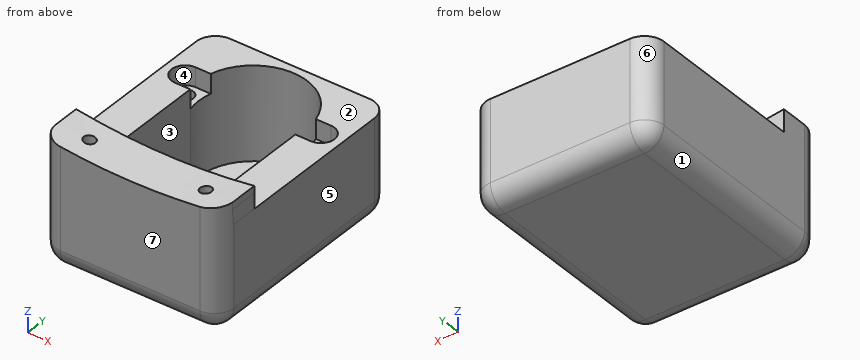
from build123d import *

# Parameters (mm, degrees)
ESQUISSE1_W             = 26
ESQUISSE1_H             = 46
BOSS_EXTRU_1_DEPTH      = 10
ESQUISSE1_5_W           = 26
ESQUISSE1_5_H           = 46
BOSS_EXTRU_2_DEPTH      = 48
ESQUISSE2_R             = 14
ESQUISSE2_R_2           = 2.5
ENL_V_MAT_EXTRU_1_DEPTH = 24
ESQUISSE2_17_R          = 2.1
ENL_V_MAT_EXTRU_2_DEPTH = 5
ESQUISSE2_18_R          = 2.1
ENL_V_MAT_EXTRU_3_DEPTH = 14
BOSS_EXTRU_7_DEPTH      = 12
CONG_1_R                = 5
CONG_2_R                = 5
ESQUISSE6_R             = 1.5
ENL_V_MAT_EXTRU_4_DEPTH = 174


with BuildPart() as part:
    # Esquisse1 → Boss.-Extru.1 (new body)
    with BuildSketch(Plane(origin=(0, 0, 0), x_dir=(0, 0, -1), z_dir=(0, 1, 0))):
        with Locations((171, 0)):
            Rectangle(ESQUISSE1_W, ESQUISSE1_H)
    extrude(amount=BOSS_EXTRU_1_DEPTH)

    # Esquisse1<5> → Boss.-Extru.2 (add)
    with BuildSketch(Plane(origin=(0, 0, 0), x_dir=(0, 0, -1), z_dir=(0, 1, 0))):
        with Locations((171, 0)):
            Rectangle(ESQUISSE1_5_W, ESQUISSE1_5_H)
    extrude(amount=-BOSS_EXTRU_2_DEPTH)

    # Esquisse2 → Enlèv. mat.-Extru.1 (cut)
    # profile 1 of 3: a face of its own
    with BuildSketch(Plane.XY.offset(-158)):
        with Locations((0, -6)):
            Circle(ESQUISSE2_R)
        with Locations((0, 2)):
            Circle(ESQUISSE2_R_2, mode=Mode.SUBTRACT)
    # profile 2 of 3: a face of its own
    with BuildSketch(Plane.XY.offset(-158)):
        with BuildLine():
            ThreePointArc((13.555441712, -9.5), (0, -20), (-13.555441712, -9.5))
            Line((-13.555441712, -9.5), (-13.555441712, -36))
            Line((-13.555441712, -36), (13.555441712, -36))
            Line((13.555441712, -36), (13.555441712, -9.5))
        make_face()
    # profile 3 of 3: a face of its own
    with BuildSketch(Plane.XY.offset(-158)):
        with Locations((0, 2)):
            Circle(ESQUISSE2_R_2)
    extrude(amount=-ENL_V_MAT_EXTRU_1_DEPTH, mode=Mode.SUBTRACT)

    # Esquisse2<17> → Enlèv. mat.-Extru.2 (cut)
    # profile 1 of 2: a face of its own
    with BuildSketch(Plane.XY.offset(-158)):
        with BuildLine():
            Line((-13.555441712, -2.5), (-17.5, -2.5))
            ThreePointArc((-17.5, -2.5), (-21, -6), (-17.5, -9.5))
            Line((-17.5, -9.5), (-13.555441712, -9.5))
            ThreePointArc((-13.555441712, -9.5), (-14, -6), (-13.555441712, -2.5))
        make_face()
        with Locations((-17.5, -6)):
            Circle(ESQUISSE2_17_R, mode=Mode.SUBTRACT)
    # profile 2 of 2: a face of its own
    with BuildSketch(Plane.XY.offset(-158)):
        with BuildLine():
            Line((17.5, -2.5), (13.555441712, -2.5))
            ThreePointArc((13.555441712, -2.5), (13.888415748, -4.235939905), (14, -6))
            ThreePointArc((14, -6), (13.888415748, -7.764060095), (13.555441712, -9.5))
            Line((13.555441712, -9.5), (17.5, -9.5))
            ThreePointArc((17.5, -9.5), (21, -6), (17.5, -2.5))
        make_face()
        with Locations((17.5, -6)):
            Circle(ESQUISSE2_17_R, mode=Mode.SUBTRACT)
    extrude(amount=-ENL_V_MAT_EXTRU_2_DEPTH, mode=Mode.SUBTRACT)

    # Esquisse2<18> → Enlèv. mat.-Extru.3 (cut)
    with BuildSketch(Plane.XY.offset(-158)):
        with Locations((-17.5, -6)):
            Circle(ESQUISSE2_18_R)
        with Locations((17.5, -6)):
            Circle(ESQUISSE2_18_R)
    extrude(amount=-ENL_V_MAT_EXTRU_3_DEPTH, mode=Mode.SUBTRACT)

    # Esquisse5 → Boss.-Extru.7 (add)
    with BuildSketch(Plane.XZ.offset(48)):
        with BuildLine():
            Line((-23, -158), (-23, -154))
            Line((-23, -154), (-23, -152.249792013))
            ThreePointArc((-23, -152.249792013), (-0.012314253, -153.999999501), (22.975654778, -152.253516723))
            Line((22.975654778, -152.253516723), (22.975654778, -154))
            Line((22.975654778, -154), (23, -158))
            Line((23, -158), (23, -184))
            Line((23, -184), (-23, -184))
            Line((-23, -184), (-23, -158))
        make_face()
    extrude(amount=-BOSS_EXTRU_7_DEPTH)

    # Congé1
    cong_1_edges = [part.edges().sort_by_distance(p)[0] for p in [
        (23, 10, -171),
        (0, 10, -184),
        (23, -19, -184),
    ]]
    fillet(cong_1_edges, radius=CONG_1_R)

    # Congé2
    # the kernel refuses this fillet: 5 mm, written as the material it takes off along each edge
    with BuildSketch(Plane(origin=(-18, -43, -179), x_dir=(-1, 0, 0), z_dir=(0, -1, 0))) as cong_2_piece_1_section:
        Polygon((0, 0), (CONG_2_R * 1.02, 0), (CONG_2_R * 1.02, CONG_2_R * 1.02), (0, CONG_2_R * 1.02), align=None)
    cong_2_piece_1 = extrude(amount=CONG_2_R * 1.02, mode=Mode.PRIVATE)
    cong_2_piece_1 = cong_2_piece_1 - Plane(origin=(-18, -43, -179), x_dir=(0.7071067811865475, 0, 0.7071067811865475), z_dir=(0, -1, 0)) * Sphere(CONG_2_R, mode=Mode.PRIVATE)
    add(cong_2_piece_1, mode=Mode.SUBTRACT)
    with BuildSketch(Plane(origin=(18, -48, -179), x_dir=(0, 0, -1), z_dir=(-1, 0, 0))) as cong_2_piece_2:
        with BuildLine():
            CenterArc((5 - CONG_2_R, -CONG_2_R), CONG_2_R, 0, 90)
            Line((5 - CONG_2_R, 0), (5, 0))
            Line((5, 0), (5, -CONG_2_R))
        make_face()
    revolve(axis=Axis((18, -48, -179), (0, -1, 0)), revolution_arc=90, mode=Mode.SUBTRACT)
    with BuildSketch(Plane(origin=(-23, 5, -179), x_dir=(0, 1, 0), z_dir=(0, 0, 1))) as cong_2_piece_3:
        with BuildLine():
            CenterArc((5 - CONG_2_R, -CONG_2_R), CONG_2_R, 0, 90)
            Line((5, -CONG_2_R), (5, 0))
            Line((5, 0), (5 - CONG_2_R, 0))
        make_face()
    revolve(axis=Axis((-23, 5, -179), (-1, 0, 0)), revolution_arc=90, mode=Mode.SUBTRACT)
    with BuildSketch(Plane(origin=(-23, -48, -179), x_dir=(0, 1, 0), z_dir=(0, 0, 1))) as cong_2_piece_4:
        with BuildLine():
            CenterArc((CONG_2_R, -CONG_2_R), CONG_2_R, 90, 90)
            Line((0, -CONG_2_R), (0, 0))
            Line((0, 0), (CONG_2_R, 0))
        make_face()
    extrude(amount=39.250207987, mode=Mode.SUBTRACT)
    with BuildSketch(Plane(origin=(23, -48, -145.5), x_dir=(0, 1, 0), z_dir=(0, 0, -1)), Plane(origin=(-23, 10, -179), x_dir=(1, 0, 0), z_dir=(0, 0, 1))) as cong_2_piece_5:
        with BuildLine():
            CenterArc((CONG_2_R, -CONG_2_R), CONG_2_R, 90, 90)
            Line((0, -CONG_2_R), (0, 0))
            Line((0, 0), (CONG_2_R, 0))
        make_face()
    extrude(amount=33.5, mode=Mode.SUBTRACT)
    with BuildSketch(Plane(origin=(18, -48, -184), x_dir=(0, 0, 1), z_dir=(-1, 0, 0))) as cong_2_piece_6:
        with BuildLine():
            CenterArc((CONG_2_R, CONG_2_R), CONG_2_R, 180, 90)
            Line((0, CONG_2_R), (0, 0))
            Line((0, 0), (CONG_2_R, 0))
        make_face()
    extrude(amount=36, mode=Mode.SUBTRACT)
    with BuildSketch(Plane(origin=(-23, 5, -184), x_dir=(0, 0, 1), z_dir=(0, -1, 0))) as cong_2_piece_7:
        with BuildLine():
            CenterArc((CONG_2_R, -CONG_2_R), CONG_2_R, 90, 90)
            Line((0, -CONG_2_R), (0, 0))
            Line((0, 0), (CONG_2_R, 0))
        make_face()
    extrude(amount=48, mode=Mode.SUBTRACT)

    # Esquisse6 → Enlèv. mat.-Extru.4 (cut)
    with BuildSketch(Plane.XY):
        with Locations((-15, -42)):
            Circle(ESQUISSE6_R)
        with Locations((15, -42)):
            Circle(ESQUISSE6_R)
    extrude(amount=-ENL_V_MAT_EXTRU_4_DEPTH, mode=Mode.SUBTRACT)


solid = part.part
Could you check a few things on this model? Use its own coordinates, in mm. Face numbers are marked on the shaded views. A direction names the side the tool comes from. Coordinates: 2 decimals unless noted, no trailing zeros. Loops run counter-clockwise (first coordinate to the right, second up) from the corner with the lowest first, then second, coordinate; pieces in that order, holes last.
1. Imagine slicing it at D-D (x = 0). Please give me the cut outline in (y, z), and give its area (3 significant figures).
2. Imagine slicing it at A-A (z = -160). Please give me the cut outline in (x, y), and give its area (3 significant figures).
3. Imagine slicing it at B-B (y = -21). Please give me the cut outline in (x, z).
4. Imagine slicing it at C-C (z = -178). Please give me the cut outline in (x, y).
5. For the marked faces 1, 2 and 3, which set-ups out of +Z, -Z, +X, -X, +Y, -Y let a thin tool reach every point of the face, with its end or its side?
6. For P1, Ø22.5, axis at x = -3.5, y = -9.5, coming from the +Z side; P2, Ø2.5, axis at x = -15.5, y = -42, coming from the +Z side; P3, Ø5.5, axis at x = 17.5, y = -6, coming from the +Z side, each with a flat end and sliding along its axis, tell me the tip position at first contact or that it passes through.
7. We'd pull the mould along X, two halves only. Please class the marked faces 4, 5, 6 and 7: released by +X, released by -X, zero draft, split by the parting line, or undercut.
8. I need wall thicknesses on L1, parallel to X at y = -42, z = -158.25; L2, parallel to Y at x = -15, z = -162.25; L3, parallel to X at y = -6, z = -175. Which ranges of each line are inside material? Lowest first, please.
Computed values:
1. outline: (-48, -179) arc R5 ccw to (-43, -184) - (5, -184) arc R5 ccw to (10, -179) - (10, -158) - (8, -158) - (8, -182) - (-36, -182) - (-36, -154) - (-48, -154) - close
1. area: 489 mm2
2. outline: (-23, -43) arc R5 ccw to (-18, -48) - (18, -48) arc R5 ccw to (23, -43) - (23, 5) arc R5 ccw to (18, 10) - (-18, 10) arc R5 ccw to (-23, 5) - close; hole (-17.5, -9.5) - (-13.56, -9.5) - (-13.56, -36) - (13.56, -36) - (13.56, -9.5) - (17.5, -9.5) arc R3.5 ccw to (17.5, -2.5) - (13.56, -2.5) arc R14 ccw to (-13.56, -2.5) - (-17.5, -2.5) arc R3.5 ccw to start; hole circle Ø3 at (-15, -42); hole circle Ø3 at (15, -42)
2. area: 1,420 mm2
3. outline: (-23, -179) arc R5 ccw to (-18, -184) - (18, -184) arc R5 ccw to (23, -179) - (23, -158) - (13.56, -158) - (13.56, -182) - (-13.56, -182) - (-13.56, -158) - (-23, -158) - close
4. outline: (-23, -43) arc R5 ccw to (-18, -48) - (18, -48) arc R5 ccw to (23, -43) - (23, 5) arc R5 ccw to (18, 10) - (-18, 10) arc R5 ccw to (-23, 5) - close; hole (-13.56, -36) - (13.56, -36) - (13.56, -9.5) arc R14 ccw (long way) to (-13.56, -9.5) - close
5. face 1: -Z, -X, +Y, -Y
5. face 2: +Z, +X, -X, +Y
5. face 3: +Z
6. P1: stops at z = -158
6. P2: stops at z = -153.07
6. P3: stops at z = -163
7. face 4: undercut
7. face 5: released by +X
7. face 6: released by -X
7. face 7: zero draft
8. L1: x = -23 to -16.5, -13.5 to 13.5, 16.5 to 23
8. L2: y = -48 to -43.5, -40.5 to -9.5, -2.5 to 10
8. L3: x = -23 to -14, 14 to 23
